Build history of the part. All positions in model axes, mm. Round coordinates to 2 decimals unless told otherwise and drop trailing zeros. Order: outer loops, then holes, each group sorted by start corner. A loop starts at its lowest first (then second) coordinate and runs counter-clockwise, first axis right, second up. Notation, with made-up numbers: (31, -21.5) -> (37, -21.5) arc R38 cw to (37, 17.5) -> close; hole circle Ø10 at (57, 17.5). An arc over 180 degrees is marked (long way). Answer as CSV lines item,"result". Start each with the question number.
```python
from build123d import *

# Parameters (mm, degrees)
SKETCH1_W           = 475
SKETCH1_H           = 356.34
BOSS_EXTRUDE1_DEPTH = 50.8
FILLET2_R           = 20
FILLET6_R           = 20
FILLET7_R           = 20


with BuildPart() as part:
    # Sketch1 → Boss-Extrude1 (new body)
    with BuildSketch(Plane.XY):
        with Locations((-51.338268793, -107.61191344)):
            Rectangle(SKETCH1_W, SKETCH1_H)
    extrude(amount=BOSS_EXTRUDE1_DEPTH)

    # Fillet2
    fillet2_edges = [part.edges().sort_by_distance(p)[0] for p in [
        (186.161731207, -107.61191344, 50.8),
        (-51.338268793, 70.55808656, 50.8),
        (-288.838268793, -107.61191344, 50.8),
        (-51.338268793, -285.78191344, 50.8),
    ]]
    fillet(fillet2_edges, radius=FILLET2_R)

    # Fillet6
    # the kernel refuses this fillet: 20 mm, written as the material it takes off along each edge
    with BuildSketch(Plane(origin=(166.161731207, 50.55808656, 30.8), x_dir=(1, 0, 0), z_dir=(0, 1, 0))) as fillet6_piece_1_section:
        Polygon((0, 0), (FILLET6_R * 1.02, 0), (FILLET6_R * 1.02, -FILLET6_R * 1.02), (0, -FILLET6_R * 1.02), align=None)
    fillet6_piece_1 = extrude(amount=FILLET6_R * 1.02, mode=Mode.PRIVATE)
    fillet6_piece_1 = fillet6_piece_1 - Plane(origin=(166.161731207, 50.55808656, 30.8), x_dir=(-0.7071067811865475, 0, -0.7071067811865475), z_dir=(0, 1, 0)) * Sphere(FILLET6_R, mode=Mode.PRIVATE)
    add(fillet6_piece_1, mode=Mode.SUBTRACT)
    with BuildSketch(Plane(origin=(166.161731207, -265.78191344, 30.8), x_dir=(0, -1, 0), z_dir=(1, 0, 0))) as fillet6_piece_2_section:
        Polygon((0, 0), (FILLET6_R * 1.02, 0), (FILLET6_R * 1.02, -FILLET6_R * 1.02), (0, -FILLET6_R * 1.02), align=None)
    fillet6_piece_2 = extrude(amount=FILLET6_R * 1.02, mode=Mode.PRIVATE)
    fillet6_piece_2 = fillet6_piece_2 - Plane(origin=(166.161731207, -265.78191344, 30.8), x_dir=(0, 0.7071067811865475, -0.7071067811865475), z_dir=(1, 0, 0)) * Sphere(FILLET6_R, mode=Mode.PRIVATE)
    add(fillet6_piece_2, mode=Mode.SUBTRACT)
    with BuildSketch(Plane(origin=(-268.838268793, 50.55808656, 30.8), x_dir=(-1, 0, 0), z_dir=(0, 1, 0))) as fillet6_piece_3_section:
        Polygon((0, 0), (FILLET6_R * 1.02, 0), (FILLET6_R * 1.02, FILLET6_R * 1.02), (0, FILLET6_R * 1.02), align=None)
    fillet6_piece_3 = extrude(amount=FILLET6_R * 1.02, mode=Mode.PRIVATE)
    fillet6_piece_3 = fillet6_piece_3 - Plane(origin=(-268.838268793, 50.55808656, 30.8), x_dir=(0.7071067811865475, 0, -0.7071067811865475), z_dir=(0, 1, 0)) * Sphere(FILLET6_R, mode=Mode.PRIVATE)
    add(fillet6_piece_3, mode=Mode.SUBTRACT)
    with BuildSketch(Plane(origin=(-268.838268793, -265.78191344, 30.8), x_dir=(0, -1, 0), z_dir=(-1, 0, 0))) as fillet6_piece_4_section:
        Polygon((0, 0), (FILLET6_R * 1.02, 0), (FILLET6_R * 1.02, FILLET6_R * 1.02), (0, FILLET6_R * 1.02), align=None)
    fillet6_piece_4 = extrude(amount=FILLET6_R * 1.02, mode=Mode.PRIVATE)
    fillet6_piece_4 = fillet6_piece_4 - Plane(origin=(-268.838268793, -265.78191344, 30.8), x_dir=(0, 0.7071067811865475, -0.7071067811865475), z_dir=(-1, 0, 0)) * Sphere(FILLET6_R, mode=Mode.PRIVATE)
    add(fillet6_piece_4, mode=Mode.SUBTRACT)
    with BuildSketch(Plane(origin=(-288.838268793, -285.78191344, -50), x_dir=(0, 1, 0), z_dir=(0, 0, 1)), Plane(origin=(-288.838268793, 70.55808656, -50), x_dir=(1, 0, 0), z_dir=(0, 0, 1))) as fillet6_piece_5:
        with BuildLine():
            CenterArc((FILLET6_R, -FILLET6_R), FILLET6_R, 90, 90)
            Line((0, -FILLET6_R), (0, 0))
            Line((0, 0), (FILLET6_R, 0))
        make_face()
    extrude(amount=80.8, mode=Mode.SUBTRACT)
    with BuildSketch(Plane(origin=(186.161731207, -285.78191344, -50), x_dir=(0, 1, 0), z_dir=(0, 0, 1)), Plane(origin=(186.161731207, 70.55808656, -50), x_dir=(-1, 0, 0), z_dir=(0, 0, 1))) as fillet6_piece_6:
        with BuildLine():
            CenterArc((FILLET6_R, FILLET6_R), FILLET6_R, 180, 90)
            Line((0, FILLET6_R), (0, 0))
            Line((0, 0), (FILLET6_R, 0))
        make_face()
    extrude(amount=80.8, mode=Mode.SUBTRACT)

    # Fillet7
    fillet7_edges = [part.edges().sort_by_distance(p)[0] for p in [
        (-51.338268793, 70.55808656, 0),
        (-288.838268793, -107.61191344, 0),
        (186.161731207, -107.61191344, 0),
        (-51.338268793, -285.78191344, 0),
        (-282.980404416, 64.700222184, 0),
        (-282.980404416, -279.924049063, 0),
        (180.303866831, -279.924049063, 0),
        (180.303866831, 64.700222184, 0),
    ]]
    fillet(fillet7_edges, radius=FILLET7_R)


solid = part.part
```
Q1. Slice it at B-B, the plane z = 41.5. Write the cut outline in (x, y), plus the area to 3 significant figures.
Q2. Probe L1, parallel to Y at x = -127.5, z = 18; L2, parallel to X at y = -48.5, z = 18; L3, parallel to X at y = -72.5, z = 31.5. List the from-to ranges inside material, lowest first.
Q3. Slice it at A-A, the plane x = -81.5. Write the cut outline in (y, z), plus the area to 3 significant figures.
Q4. Flat gauge pins, fed straight in: pin 1 Ø12 at (x, z) = (-35, 9.5) entering from +Y; pin 2 Ø1.5 at (x, z) = (52, 15) entering from -Y. Where does each tip first touch, or does it go through?
Solutions:
1,outline,"(-285.74, -265.78) arc R16.9 ccw to (-268.84, -282.68) -> (166.16, -282.68) arc R16.9 ccw to (183.06, -265.78) -> (183.06, 50.56) arc R16.9 ccw to (166.16, 67.46) -> (-268.84, 67.46) arc R16.9 ccw to (-285.74, 50.56) -> close"
1,area,"164,000 mm2"
2,L1,"y = -285.68 to 70.46"
2,L2,"x = -288.74 to 186.06"
2,L3,"x = -288.83 to 186.15"
3,outline,"(-285.78, 20) arc R20 ccw to (-265.78, 0) -> (50.56, 0) arc R20 ccw to (70.56, 20) -> (70.56, 30.8) arc R20 ccw to (50.56, 50.8) -> (-265.78, 50.8) arc R20 ccw to (-285.78, 30.8) -> close"
3,area,"17,800 mm2"
4,pin 1,"stops at y = 70.05"
4,pin 2,"stops at y = -285.33"
